```python
from build123d import *

# Parameters (mm, degrees)
F0_W     = 101.6
F0_H     = 101.6
F1_DEPTH = 101.6
F2_R     = 25.4
F3_DEPTH = 203.2
F6_W     = 50.8
F6_H     = 50.8
F7_DEPTH = 101.6
F8_R     = 6.35


with BuildPart() as f1:
    # F0 (on Top) → F1 (new body)
    with BuildSketch(Plane.XY):
        Rectangle(F0_W, F0_H)
    extrude(amount=F1_DEPTH)

    # F2 (on Top) → F3 (join)
    with BuildSketch(Plane.XY):
        Circle(F2_R)
    extrude(amount=F3_DEPTH)

    # F4 (on face) → F5 (revolve)
    with BuildSketch(Plane.XY.offset(203.2)):
        with BuildLine():
            Line((0, -25.4), (0, -38.1))
            ThreePointArc((0, -38.1), (38.1, 0), (0, 38.1))
            Line((0, 38.1), (0, 25.4))
            ThreePointArc((0, 25.4), (17.9605122421, 17.9605122421), (25.4, 0))
            ThreePointArc((25.4, 0), (17.9605122421, -17.9605122421), (0, -25.4))
        make_face()
        with BuildLine():
            Line((0, 25.4), (0, -25.4))
            ThreePointArc((0, -25.4), (17.9605122421, -17.9605122421), (25.4, 0))
            ThreePointArc((25.4, 0), (17.9605122421, 17.9605122421), (0, 25.4))
        make_face()
    revolve(axis=Axis((0, 0, 203.2), (0, -1, 0)))

    # F6 (on face) → F7 (cut)
    with BuildSketch(Plane.XZ.offset(50.8)):
        with Locations((0, 50.8)):
            Rectangle(F6_W, F6_H)
    extrude(amount=-F7_DEPTH, mode=Mode.SUBTRACT)

    # F8
    f8_edges = [f1.edges().sort_by_distance(p)[0] for p in [
        (-25.4, 0, 101.6),
        (50.8, 0, 101.6),
        (50.8, -50.8, 50.8),
        (0, -50.8, 101.6),
        (0, 50.8, 101.6),
        (-50.8, 0, 101.6),
        (-25.4, 0, 174.801937),
        (50.8, 50.8, 50.8),
        (50.8, 0, 0),
        (0, -50.8, 0),
        (-50.8, -50.8, 50.8),
        (-50.8, 50.8, 50.8),
        (0, 50.8, 0),
        (-50.8, 0, 0),
    ]]
    fillet(f8_edges, radius=F8_R)


solid = f1.part
```
Source: CAD feature listing. Evaluate the final solid. Frame: model axes, mm. A direction names the side the tool comes from. Coordinates: 2 decimals unless noted, no trailing zeros. Loops run counter-clockwise (first coordinate to the right, second up) from the corner with the lowest first, then second, coordinate; pieces in that order, holes last. Notation, with made-up numbers: (39.5, -36) -> (93.5, -36) arc R19 cw to (93.5, -10) -> close; hole circle Ø6 at (31, -18). An arc over 180 degrees is marked (long way). One line per item, written item: value. Start each with the question number.
Q1. Line query: line 1 along X through (y, z) = (-14, 54.5); line 2 along Z through (x, y) = (-17, -24); line 3 along Z through (x, y) = (17, 28). Output: solid intervals per line, ascending.
Q2. Section query A-A, the plane z = 120. Return the cut outline in (x, y).
Q3. Contact query for flat-ended pins moving along their axis: P1, Ø6, axis at x = -15, y = 27, coming from the +Z side; P2, Ø3, axis at x = -18.5, z = 152.5, coming from the +Y side; P3, Ø10, axis at x = 3.5, z = 161.5, coming from the -Y side. Output: stop coordinate, or through.
Q4. Section query B-B, the plane z = 194.5. Return the cut outline in (x, y), and give its area (3 significant figures).
Q5. Mould query, pull axis X, two halves, no side actions, for faces 1 (the face through (0, -1, 25.4)), 2 (the face through (0.62, -48.99, 1.91)), 3 (the face through (48.89, 0.62, 99.79)). Classes: pulls with the +X half, pulls with the -X half, needs draft (parallel to the pull), parting line crosses it, or undercut.
Q6. Set-up query: faces 4 (the face through (-50.8, -1, 50)), 5 (the face through (0, -1, 76.2)), 6 (the face through (-11, 30, 101.6)). Return all of +Z, -Z, +X, -X, +Y, -Y with unobstructed straight access to the full face (end or side cutting, diameter ignored); none if empty.
Results:
1. line 1: -50.8 to -25.4, 25.4 to 50.8
1. line 2: 0 to 25.4, 76.2 to 102.05, 178.98 to 227.42
1. line 3: 0 to 25.4, 76.2 to 101.6, 183.74 to 222.66
2. outline: circle Ø50.8 at (0, 0)
3. P1: z = 229.16
3. P2: y = 18.87
3. P3: y = -25.4
4. outline: circle Ø74.19 at (0, 0)
4. area: 4,320 mm^2
5. face 1: undercut
5. face 2: needs draft
5. face 3: pulls with the +X half
6. face 4: +Z, -Z, -X, +Y, -Y
6. face 5: +Y, -Y
6. face 6: none
